Verification items for the finished model (mm, model axes). Round coordinates to 2 decimals unless told otherwise and drop trailing zeros. Loops run counter-clockwise (first coordinate to the right, second up) from the corner with the lowest first, then second, coordinate; pieces in that order, holes last. Notation, with made-up numbers: (-27, 64) - (9, 64) arc R28 ccw to (9, 93) - close; hole circle Ø11 at (43.25, -27.5). An arc over 180 degrees is marked (long way). Use CSV: the item, a comma, the result in double quotes.
```python
from build123d import *

# Parameters (mm, degrees)
BOSS_EXTRUDE1_DEPTH      = 180
BOSS_EXTRUDE1_DEPTH_BACK = 180
SKETCH1_W                = 10
SKETCH1_H                = 10
SKETCH1_R                = 4
FILLET1_R                = 1


with BuildPart() as part:
    # Sketch1 → Boss-Extrude1 (new, two sides: drawn at the far end of the back side and taken through both)
    with BuildSketch(Plane.XY.offset(-BOSS_EXTRUDE1_DEPTH_BACK)):
        Rectangle(SKETCH1_W, SKETCH1_H)
        Circle(SKETCH1_R, mode=Mode.SUBTRACT)
    extrude(amount=BOSS_EXTRUDE1_DEPTH + BOSS_EXTRUDE1_DEPTH_BACK)

    # Fillet1
    fillet1_edges = [part.edges().sort_by_distance(p)[0] for p in [
        (-5, 5, 0),
        (5, 5, 0),
        (5, -5, 0),
        (-5, -5, 0),
    ]]
    fillet(fillet1_edges, radius=FILLET1_R)


solid = part.part
```
1) Mould release check, pull along Y, two halves, no side actions. Record for faces 1 (the face through (-0.867, -3.905, -2.52)), 2 (the face through (5, 0, -3)), 3 (the face through (0, -5, -3)): +Y half, -Y half, draft (parallel to the pull), parting line (faces both ways), or undercut.
Returned:
face 1,"undercut"
face 2,"draft"
face 3,"-Y half"
2) Thickness scan on probe 1 along Y at (x, z) = (0, 81); probe 2 along Y at (x, z) = (-0.75, 155); probe 3 along X at (y, z) = (-0.5, 38). Record the ranges inside material, lowest first. Write a range as [from, to].
Returned:
probe 1,"y = [-5, -4], [4, 5]"
probe 2,"y = [-5, -3.93], [3.93, 5]"
probe 3,"x = [-5, -3.97], [3.97, 5]"
3) Cross-section at A-A, the plane x = 0. Record the cut outline in (y, z).
Returned:
outline,"(-5, -180) - (-4, -180) - (-4, 180) - (-5, 180) - close; (4, -180) - (5, -180) - (5, 180) - (4, 180) - close"
4) Cross-section at C-C, the plane z = -40. Record the cut outline in (x, y), then the cut area to 3 significant figures.
Returned:
outline,"(-5, -4) arc R1 ccw to (-4, -5) - (4, -5) arc R1 ccw to (5, -4) - (5, 4) arc R1 ccw to (4, 5) - (-4, 5) arc R1 ccw to (-5, 4) - close; hole circle Ø8 at (0, 0)"
area,"48.9 mm²"
